Job drawing, mm, ordinate dimensions from the low corner. One solid piece. A direction names the side the tool comes from. Give positions to 0.01 mm unless a question says otherwise; leave off trailing zeros. Write each loop counter-clockwise with the first axis right and the second up, starting at its lowest first coordinate (ties: lowest second). Pieces come first, ordered by that corner, then holes. Notation, with made-up numbers: (-23, 50.25) - (-10, 50.25) arc R27 ccw to (-10, 76.25) - close; hole circle Ø2 at (-22, 41). An arc over 180 degrees is marked (long way). Answer as a JSON object with one key per item and string values.
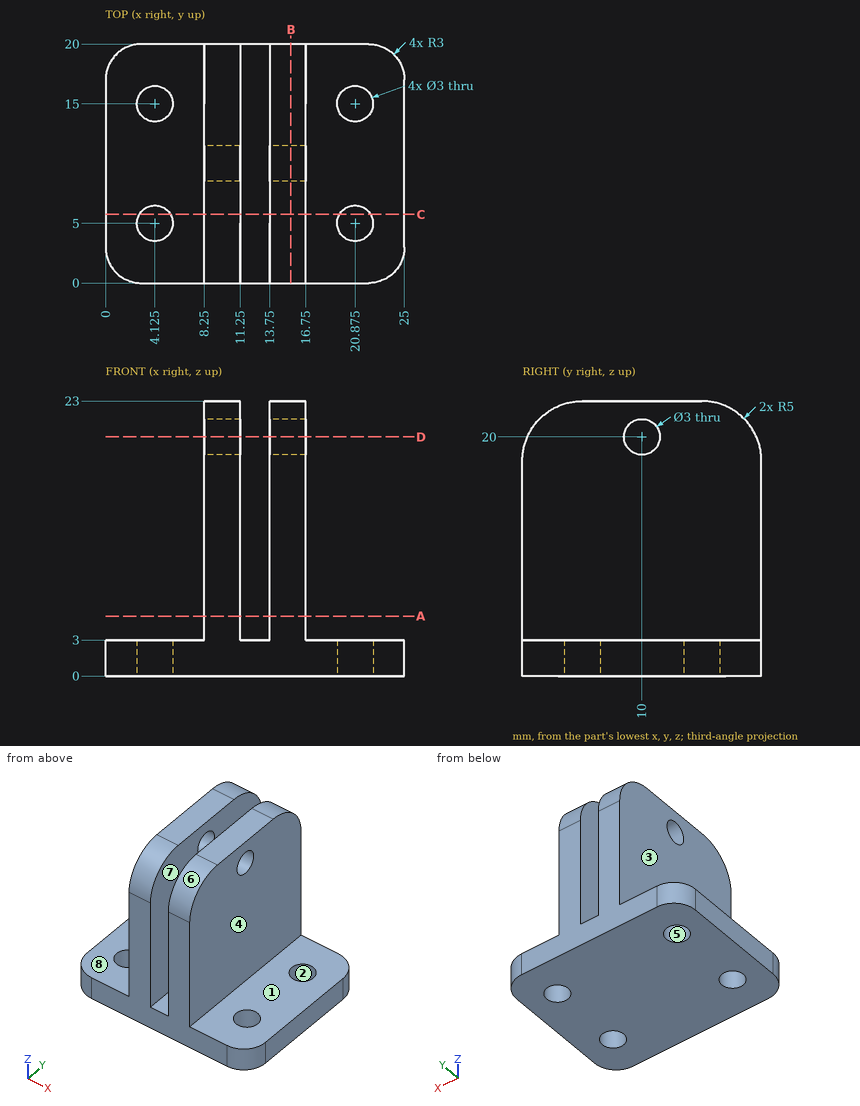
Item 1: Probe line 1 (X direction, y = 5, z = 2.1) (3 decimals); line 2 (X direction, y = 14, z = 5.5); line 3 (Z direction, x = 8, y = 13.5). List the from-to ranges inside material, lowest first. Write a range as from..to.
Entries:
{"line 1": "0..2.625, 5.625..19.375, 22.375..25", "line 2": "8.25..11.25, 13.75..16.75", "line 3": "0..3"}
Item 2: Mould opens along X. For the marked faces 1, 2 and 3 say: +X half, -X half, draft (parallel to the pull), parting line (faces both ways), or undercut.
Entries:
{"face 1": "draft", "face 2": "undercut", "face 3": "-X half"}
Item 3: Flat gauge pins, fed straight in: P1, Ø1.8, axis at y = 10, z = 20, coming from the +X side; P2, Ø0.8, axis at x = 12.5, y = 12.5, coming from the +Z side; P3, Ø6, axis at y = 9.5, z = 20, coming from the +X side; P4, Ø2, axis at y = 14, z = 10, coming from the -X side. Where does each tip first touch, or does it go through?
Entries:
{"P1": "through", "P2": "z = 3", "P3": "x = 16.75", "P4": "x = 8.25"}
Item 4: Cut at A-A (z = 5). Give the cut face in (x, y), and give its area (3 significant figures).
Entries:
{"outline": "(8.25, 0) - (11.25, 0) - (11.25, 20) - (8.25, 20) - close; (13.75, 0) - (16.75, 0) - (16.75, 20) - (13.75, 20) - close", "area": "120 mm2"}
Item 5: Which spindle directions (+Z, -Z, +X, -X, +Y, -Y) get a long thin tool onto all of the face, cutting with end or side? Do the marked faces 4, 5, 6, 7 and 8. Say none if no direction does.
Entries:
{"face 4": "+Z, +X, +Y, -Y", "face 5": "+Z, -Z", "face 6": "+Z, +X, -X, -Y", "face 7": "+Z, +Y, -Y", "face 8": "+Z, -X, +Y, -Y"}
Item 6: Cut at D-D (z = 20). Give the cut face in (x, y).
Entries:
{"outline": "(8.25, 0.42) - (11.25, 0.42) - (11.25, 8.5) - (8.25, 8.5) - close; (8.25, 11.5) - (11.25, 11.5) - (11.25, 19.58) - (8.25, 19.58) - close; (13.75, 0.42) - (16.75, 0.42) - (16.75, 8.5) - (13.75, 8.5) - close; (13.75, 11.5) - (16.75, 11.5) - (16.75, 19.58) - (13.75, 19.58) - close"}
Item 7: Cut at B-B (x = 15.5). Give the cut face in (y, z), and give its area (3 significant figures).
Entries:
{"outline": "(0, 0) - (20, 0) - (20, 18) arc R5 ccw to (15, 23) - (5, 23) arc R5 ccw to (0, 18) - close; hole circle Ø3 at (10, 20)", "area": "442 mm2"}
Item 8: Cut at C-C (y = 5.75). Give the cut face in (x, z), and give its area (3 significant figures).
Entries:
{"outline": "(0, 0) - (2.83, 0) - (2.83, 3) - (0, 3) - close; (5.42, 0) - (19.58, 0) - (19.58, 3) - (16.75, 3) - (16.75, 23) - (13.75, 23) - (13.75, 3) - (11.25, 3) - (11.25, 23) - (8.25, 23) - (8.25, 3) - (5.42, 3) - close; (22.17, 0) - (25, 0) - (25, 3) - (22.17, 3) - close", "area": "179 mm2"}
